Part model, mm, in its own coordinate system. Face numbers are marked on the shaded views. A direction names the side the tool comes from. Round coordinates to 2 decimals unless told otherwise and drop trailing zeros. Write each loop counter-clockwise with the first axis right and the second up, starting at its lowest first coordinate (ties: lowest second). Pieces come first, ordered by that corner, then holes. Notation, with made-up numbers: M 67,19 L 84,19 A28 ccw 84,41 Z; hole C -2.75,7 d8. An arc over 180 degrees is marked long. Answer as a JSON object with one key per item and string values. Group by question number.
1. Band-saw the part on A-A, the plane y = -9. Write the cut outline in (x, z), plus the area to 3 significant figures.
2. Two-plate mould, pull along X, no slides. Class the marked faces 1, 2, 3 and 4: +X half, -X half, draft (parallel to the pull), parting line (faces both ways), or undercut.
3. Which spindle directions (+Z, -Z, +X, -X, +Y, -Y) get a long thin tool onto all of the face, cutting with end or side? Do the marked faces 5, 6 and 7. Say none if no direction does.
4. Band-saw the part on B-B, the plane y = 37. Write the cut outline in (x, z).
5. Drop flat-ended pins along their axis: pin 1 (1.6 mm diameter, centred on x = 17.3, y = -18, fed in from -Z); pin 2 (1.8 mm diameter, centred on x = 1, z = 4, fed in from +Y). Give the stop position or say it passes through.
6. Band-saw the part on C-C, the plane x = -17.3. Write the cut outline in (y, z).
7. Drill centre lines: line 1 (Y direction, x = 17.3, z = 4.3); line 2 (X direction, y = -6, z = 3.7); line 3 (Y direction, x = 2, z = 2.65). Where is each one in solid material? Low to high. Write a range as from..to.
8. Band-saw the part on D-D, the plane z = 3.35. Write the cut outline in (x, y).
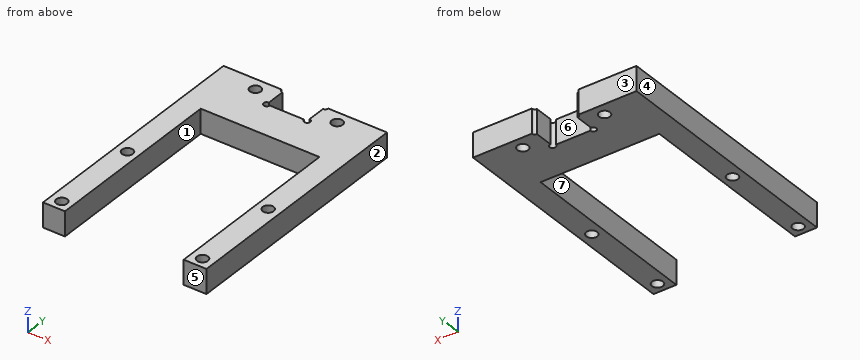
Autodesk Inventor part; units mm, degrees
ref_plane "YZ Plane" through (0, 0, 0) normal (1, 0, 0) x (0, 1, 0)
ref_plane "XZ Plane" through (0, 0, 0) normal (0, 1, 0) x (-1, 0, 0)
ref_plane "XY Plane" through (0, 0, 0) normal (0, 0, 1) x (1, 0, 0)
ref_plane "작업 평면1" through (0, 0, 0) normal (0, 0, 1) x (1, 0, 0)
sketch "스케치1" plane through (0, 0, 0) normal (0, 0, 1) x (1, 0, 0)
  line L0 (14.5, -41) -> (14.5, 11)
  line L1 (20.1, -39.6766) -> (20.1, 4.5766)
  line L2 (-20.1, 4.5766) -> (-20.1, -39.6766)
  line L3 (-14.5, 11) -> (-14.5, -41)
  circle A0 centre (-17.3, -18) radius 1.35
  circle A1 centre (17.3, -18) radius 1.35
  circle A2 centre (17.3, 4) radius 1.35
  circle A3 centre (-17.3, 4) radius 1.35
  circle A4 centre (17.3, -18) radius 1.45
  circle A5 centre (-17.3, -18) radius 1.45
  circle A6 centre (-17.3, 4) radius 1.45
  circle A7 centre (17.3, 4) radius 1.45
  line L4 (14.7, -41) -> (14.7, 11)
  line L5 (-14.7, 11) -> (-14.7, -41)
  line L6 (20.1, -20.5011) -> (-20.1, -20.5011)
  line L7 (-20.1, 0) -> (-20.1, 40)
  line L8 (20.1, -20.5011) -> (20.1, 40)
  line L9 (20.1, 40) -> (-20.1, 40)
  line L10 (14.5, 0) -> (14.5, 25)
  line L11 (14.5, 25) -> (-14.7, 25)
  line L12 (-14.7, 25) -> (-14.7, 0)
  line L13 (20.1, 40) -> (15.1, 40)
  line L14 (20.1, 40) -> (10.05, 40)
  line L15 (10.05, 40) -> (0, 40)
  line L16 (0, 40) -> (-10.05, 40)
  line L17 (-10.05, 40) -> (-20.1, 40)
  line L18 (20.1, 25) -> (20.1, 32.5)
  circle A8 centre (10.05, 32.5) radius 1.4
  circle A9 centre (-10.05, 32.5) radius 1.4
  point P0 (0, 0)
  point P1 (0, -20.5011)
  point P2 (-14.7, -20.5011)
  point P3 (14.5, -20.5011)
  dimension "d0" = 0.1
  dimension "d1" = 0.1
  dimension "d2" = -0.1
  dimension "d3" = 0.1
  dimension "d4" = 0.2
  dimension "d5" = 0.2
  dimension "d6" = 20.5011
  dimension "d7" = 40
  dimension "d9" = 15
  dimension "d12" = 5
  dimension "d13" = 40.2
  dimension "d14" = 10.05
  dimension "d15" = 10.05
  dimension "d16" = 10.05
  dimension "d17" = 10.05
  dimension "d18" = 7.5
  dimension "d19" = 2.8
  dimension "d20" = 2.8
  dimension "d21" = 20.1
extrude "돌출1" add sketch "스케치1" along normal blind 6 contours L0 L10 L11 L12 L5 L6 L2 L7 L9 L8 L1 | A4 | A5 | A6 | A7 | A8 | A9
sketch "스케치3" plane through (-20.1, 40, 0) normal (0, 1, 0) x (1, 0, 0)
  line L0 (40.2, 0) -> (0, 0)
  line L1 (0, 0) -> (0, -6)
  line L2 (40.2, -6) -> (0, -6)
  line L3 (40.2, 0) -> (40.2, -6)
  point P0 (20.1, 0)
  dimension "d29" = 40.2
sketch "스케치4" plane through (0, 0, 6) normal (0, 0, 1) x (1, 0, 0)
  line L0 (20.1, 40) -> (-20.1, 40)
  line L1 (-20.1, 40) -> (20.1, 40)
  line L2 (20.1, 40) -> (20.1, 34)
  line L3 (20.1, 34) -> (-20.1, 34)
  line L4 (-20.1, 34) -> (-20.1, 40)
  line L5 (-20.1, 40) -> (-10.05, 40)
  line L6 (-10.05, 40) -> (10.05, 40)
  circle A0 centre (-10.05, 37) radius 1.35
  circle A1 centre (10.05, 37) radius 1.35
  point P0 (0, 0)
  dimension "d30" = 6
  dimension "d31" = 10.05
  dimension "d32" = 20.1
  dimension "d33" = 2.7
  dimension "d34" = 2.7
extrude "돌출3" cut sketch "스케치4" against normal blind 10 contours A0 | A1
sketch "스케치5" plane through (0, 0, 6) normal (0, 0, 1) x (1, 0, 0)
  circle A0 centre (10.05, 37) radius 1.35
  circle A1 centre (-10.05, 37) radius 1.35
  line L0 (14.5, 25) -> (14.5, -20.5011)
  line L1 (14.5, -20.5011) -> (20.1, -20.5011)
  line L2 (20.1, -20.5011) -> (20.1, 40)
  line L3 (20.1, 40) -> (-20.1, 40)
  line L4 (-20.1, 40) -> (-20.1, -20.5011)
  line L5 (-20.1, -20.5011) -> (-14.7, -20.5011)
  line L6 (-14.7, -20.5011) -> (-14.7, 25)
  line L7 (-14.7, 25) -> (14.5, 25)
  circle A2 centre (17.3, 4) radius 1.35
  circle A3 centre (17.3, -18) radius 1.35
  circle A4 centre (-17.3, -18) radius 1.35
  circle A5 centre (-17.3, 4) radius 1.35
  line L8 (4.9, 34) -> (-5.1, 34)
  line L9 (-5.1, 34) -> (-5.1, 40)
  line L10 (-5.1, 40) -> (4.9, 40)
  line L11 (4.9, 40) -> (4.9, 34)
  line L12 (4.9, 34) -> (-5.1, 40) construction
  line L13 (-5.1, 34) -> (4.9, 40) construction
  circle A6 centre (-5.1, 40) radius 0.75
  circle A7 centre (-5.1, 34) radius 0.75
  circle A8 centre (4.9, 34) radius 0.75
  circle A9 centre (4.9, 40) radius 0.75
  point P0 (0, 0)
  point P1 (-0.1, 37)
  point P2 (4.15, 34)
  point P3 (4.9, 34.75)
  point P4 (-5.1, 34.75)
  point P5 (-4.35, 34)
  point P6 (-5.1, 39.25)
  point P7 (-4.35, 40)
  point P8 (4.9, 39.25)
  point P9 (5.65, 40)
  dimension "d37" = 10
  dimension "d40" = 1.5
  dimension "d41" = 1.5
  dimension "d42" = 1.5
  dimension "d43" = 1.5
extrude "돌출4" cut sketch "스케치5" against normal blind 6 contours A9 L11 L3 | L11 A9 L3 | A9 L11 A8 L8 A7 L9 A6 L3 | A6 L3 | L3 L9 A6 | A6 L9 L3 | A8 L8 L11 | L11 L8 A8 | A7 L8 L9 | L9 L8 A7
properties part number "feet_holder2" material "PMMA 플라스틱"
Worked answers:
{
 "1": {"outline": "M -20.1,0 L -14.7,0 L -14.7,6 L -20.1,6 Z; M 14.5,0 L 20.1,0 L 20.1,6 L 14.5,6 Z", "area": "66.0 mm^2"},
 "2": {"face 1": "undercut", "face 2": "+X half", "face 3": "draft", "face 4": "-X half"},
 "3": {"face 5": "+Z, -Z, +X, -X, -Y", "face 6": "+Z, -Z, +Y", "face 7": "+Z, -Z, -Y"},
 "4": {"outline": "M -20.1,0 L -11.4,0 L -11.4,6 L -20.1,6 Z; M -8.7,0 L -5.1,0 L -5.1,6 L -8.7,6 Z; M 4.9,0 L 8.7,0 L 8.7,6 L 4.9,6 Z; M 11.4,0 L 20.1,0 L 20.1,6 L 11.4,6 Z"},
 "5": {"pin 1": "passes through", "pin 2": "stops at y = 34"},
 "6": {"outline": "M -20.5,0 L -19.35,0 L -19.35,6 L -20.5,6 Z; M -16.65,0 L 2.65,0 L 2.65,6 L -16.65,6 Z; M 5.35,0 L 40,0 L 40,6 L 5.35,6 Z"},
 "7": {"line 1": "y = -20.5..-19.35, -16.65..2.65, 5.35..40", "line 2": "x = -20.1..-14.7, 14.5..20.1", "line 3": "y = 25..34"},
 "8": {"outline": "M -20.1,-20.5 L -14.7,-20.5 L -14.7,25 L 14.5,25 L 14.5,-20.5 L 20.1,-20.5 L 20.1,40 L 5.65,40 A0.75 cw 4.9,39.25 L 4.9,34.75 A0.75 cw long 4.15,34 L -4.35,34 A0.75 cw long -5.1,34.75 L -5.1,39.25 A0.75 cw -5.85,40 L -20.1,40 Z; hole C -17.3,-18 d2.7; hole C -17.3,4 d2.7; hole C -10.05,37 d2.7; hole C 10.05,37 d2.7; hole C 17.3,-18 d2.7; hole C 17.3,4 d2.7"}
}
